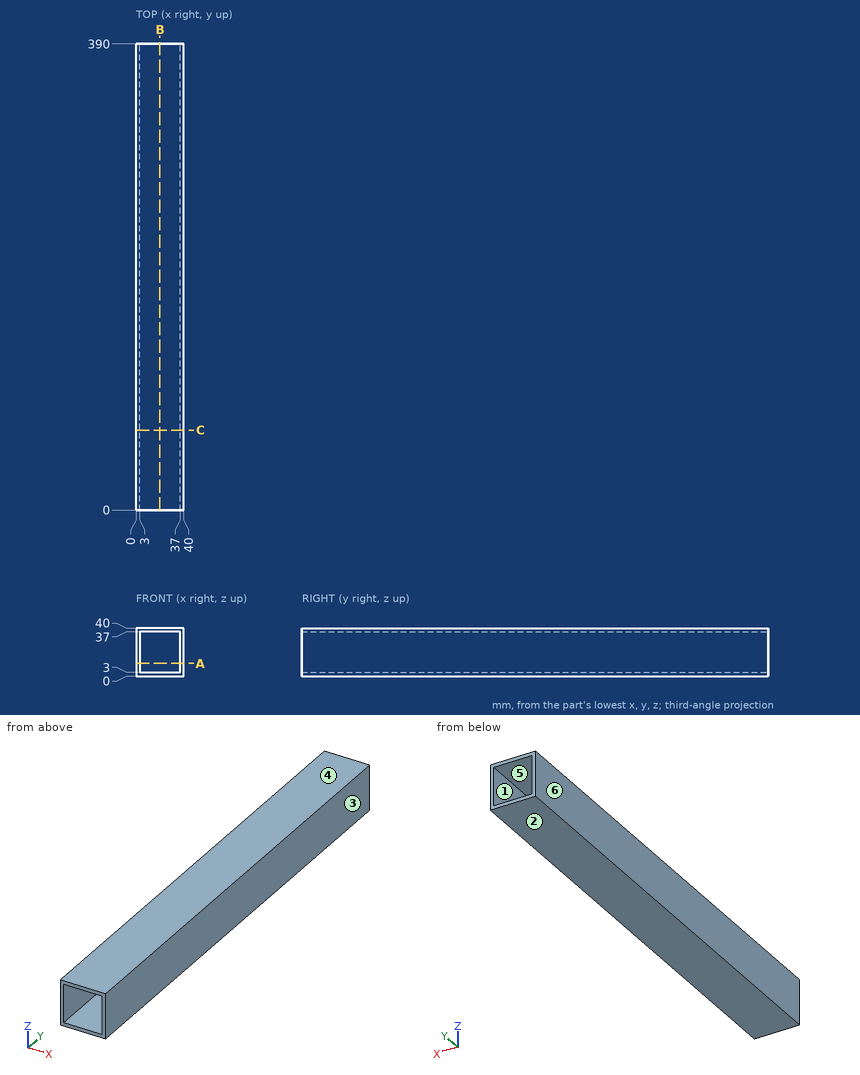
Source: three-view drawing plus pictorial views. Frame: mm from the lowest corner of the part. A direction names the side the tool comes from. Round coordinates to 2 decimals unless told otherwise and drop trailing zeros. Order: outer loops, then holes, each group sorted by start corner. A loop starts at its lowest first (then second) coordinate and runs counter-clockwise, first axis right, second up. Notation, with made-up numbers: (-22.5, 61) -> (36.5, 61) arc R16 cw to (36.5, 84) -> close; hole circle Ø9 at (28, 47). An arc over 180 degrees is marked (long way). Use CSV: the item, a comma, the result in double quotes. Start each with the question number.
1) First-contact query: pin 1 Ø8 at (x, z) = (9, 25.5) entering from -Y. Flat tip, straight axial feed; report the tip coordinate or a pass-through.
2) Material intervals for line 1 along X through (y, z) = (23.5, 26), sorted ascending. Write a range as from..to.
3) Draft query along X for the marked faces 3, 4, 5 and 6. Return one class per face: +X half, -X half, draft (parallel to the pull), parting line (faces both ways), or undercut.
4) Section A-A (z = 10.5). Return the cut outline in (x, y).
5) Section C-C (y = 67). Return the cut outline in (x, z).
6) Set-up query: the marked faces 1 and 2. Return all of +Z, -Z, +X, -X, +Y, -Y with unobstructed straight access to the full face (end or side cutting, diameter ignored); none if empty.
7) Section B-B (x = 20). Return the cut outline in (y, z).
Returned:
1,pin 1,"passes through"
2,line 1,"x = 0..3, 37..40"
3,face 3,"+X half"
3,face 4,"draft"
3,face 5,"undercut"
3,face 6,"-X half"
4,outline,"(0, 0) -> (3, 0) -> (3, 390) -> (0, 390) -> close; (37, 0) -> (40, 0) -> (40, 390) -> (37, 390) -> close"
5,outline,"(0, 0) -> (40, 0) -> (40, 40) -> (0, 40) -> close; hole (3, 3) -> (37, 3) -> (37, 37) -> (3, 37) -> close"
6,face 1,"+Y, -Y"
6,face 2,"-Z, +X, -X, +Y, -Y"
7,outline,"(0, 0) -> (390, 0) -> (390, 3) -> (0, 3) -> close; (0, 37) -> (390, 37) -> (390, 40) -> (0, 40) -> close"
